For this review, take the finished solid that the model builds, in its own axes (mm). A direction names the side the tool comes from. Round coordinates to 2 decimals unless told otherwise and drop trailing zeros. Order: outer loops, then holes, each group sorted by start corner. A loop starts at its lowest first (then second) coordinate and runs counter-clockwise, first axis right, second up. Notation, with made-up numbers: M -33,33 L -12,33 A10 cw -12,37 Z; hole C 52,84.25 d1. An arc over 180 degrees is marked long. Put each result on its own line as item: value.
from build123d import *

# Parameters (mm, degrees)
F0_W     = 109.893255
F0_H     = 54.223648
F0_W_2   = 100.012504
F0_H_2   = 45.065875
F1_DEPTH = 50.8
F2_W     = 41.578656
F2_H     = 18.166602
F4_DEPTH = 70.612
F3_R     = 7.528812
F5_DEPTH = 124.714


with BuildPart() as f1:
    # F0 (on Top) → F1 (new body)
    with BuildSketch(Plane.XY):
        with Locations((4.458386, 16.628586)):
            Rectangle(F0_W, F0_H)
        with Locations((5.060874, 16.387591)):
            Rectangle(F0_W_2, F0_H_2, mode=Mode.SUBTRACT)
    extrude(amount=F1_DEPTH)

    # F2 (on face) → F4 (cut)
    with BuildSketch(Plane.XZ.offset(10.483238)):
        with Locations((3.844391, 41.716699)):
            Rectangle(F2_W, F2_H)
    extrude(amount=-F4_DEPTH, mode=Mode.SUBTRACT)

    # F3 (on face) → F5 (cut)
    with BuildSketch(Plane.YZ.offset(59.405014)):
        with Locations((17.456431, 24.588371)):
            Circle(F3_R)
    extrude(amount=-F5_DEPTH, mode=Mode.SUBTRACT)


solid = f1.part
(1) Add section A-A on y = 33. Give the boundary of the cut face in (x, z), then the cut area to 3 significant figures.
A:
outline: M -50.49,0 L -44.95,0 L -44.95,50.8 L -50.49,50.8 Z; M 55.07,0 L 59.41,0 L 59.41,50.8 L 55.07,50.8 Z
area: 502 mm2
(2) Add section B-B on x = 48. Give the boundary of the cut face in (y, z).
A:
outline: M -10.48,0 L -6.15,0 L -6.15,50.8 L -10.48,50.8 Z; M 38.92,0 L 43.74,0 L 43.74,50.8 L 38.92,50.8 Z
(3) Add section D-D on y = 23. Give the boundary of the cut face in (x, z).
A:
outline: M -50.49,0 L -44.95,0 L -44.95,19.49 L -50.49,19.49 Z; M -50.49,29.68 L -44.95,29.68 L -44.95,50.8 L -50.49,50.8 Z; M 55.07,0 L 59.41,0 L 59.41,19.49 L 55.07,19.49 Z; M 55.07,29.68 L 59.41,29.68 L 59.41,50.8 L 55.07,50.8 Z
(4) Add section C-C on z = 38. Give the boundary of the cut face in (x, y).
A:
outline: M -50.49,-10.48 L -16.94,-10.48 L -16.94,-6.15 L -44.95,-6.15 L -44.95,38.92 L -16.94,38.92 L -16.94,43.74 L -50.49,43.74 Z; M 24.63,-10.48 L 59.41,-10.48 L 59.41,43.74 L 24.63,43.74 L 24.63,38.92 L 55.07,38.92 L 55.07,-6.15 L 24.63,-6.15 Z
(5) Draft analysis for pull direction Y (two halves, no side actions). For faces 1 (the face through (4, 43.74, 25)), 2 (the face through (4, -6.145, 25)), 3 (the face through (56, 19, 50.8)), state which applies: released by +Y, released by -Y, zero draft, split by the parting line, or undercut.
A:
face 1: released by +Y
face 2: undercut
face 3: zero draft
(6) To check wall thickness, follow L1, parallel to X at y = 25, z = 42.5; L2, parallel to Y at x = -33.5, z = 26; L3, parallel to X at y = -8, z = 45. State the ranges of each line that lie inside material, in increasing order.
A:
L1: x = -50.49 to -44.95, 55.07 to 59.41
L2: y = -10.48 to -6.15, 38.92 to 43.74
L3: x = -50.49 to -16.94, 24.63 to 59.41
(7) For faces 4 (the face through (-16.945, -8, 42)), 5 (the face through (59.405, 10, 31)), 6 (the face through (-44.945, 11, 31)), list the 3-axis set-ups (+Z, -Z, +X, -X, +Y, -Y) from which the entire face can be reached by the end or side of a thin tool; tool diameter is ignored.
A:
face 4: +Z, +Y, -Y
face 5: +Z, -Z, +X, +Y, -Y
face 6: +Z, -Z
(8) Insertion check: pin 1 Ø1.3 at (x, y) = (-5.5, -8) entering from +Z; pin 2 Ø2 at (x, y) = (21.5, 37) entering from -Z. Each pin has a flat end and moves straight along its axis. Give the tip position at first contact, or say it passes through.
A:
pin 1: stops at z = 32.63
pin 2: passes through
